Geometry: final body of the model. Coordinates: model frame, mm. A direction names the side the tool comes from. Round coordinates to 2 decimals unless told otherwise and drop trailing zeros. Loops run counter-clockwise (first coordinate to the right, second up) from the corner with the lowest first, then second, coordinate; pieces in that order, holes last. Notation, with made-up numbers: (46, -35) - (82, -35) arc R10 cw to (82, -22) - close; hole circle Ø3 at (-24.75, -37). An arc over 180 degrees is marked (long way). Answer as CSV lines item,"result".
from build123d import *

# Parameters (mm, degrees)
CROQUIS1_W              = 65
CROQUIS1_H              = 19.5
SALIENTE_EXTRUIR1_DEPTH = 16
CORTAR_EXTRUIR1_DEPTH   = 16
REDONDEO1_R             = 5
CROQUIS4_W              = 65
CROQUIS4_H              = 1.7
CORTAR_EXTRUIR2_DEPTH   = 0.57


with BuildPart() as part:
    # Croquis1 → Saliente-Extruir1 (new body)
    with BuildSketch(Plane(origin=(0, 0, 0), x_dir=(1, 0, 0), z_dir=(0, 1, 0))):
        with Locations((5.631188119, 0.14480198)):
            Rectangle(CROQUIS1_W, CROQUIS1_H)
    extrude(amount=SALIENTE_EXTRUIR1_DEPTH)

    # Croquis2 → Cortar-Extruir1 (cut)
    with BuildSketch(Plane(origin=(0, 16, 0), x_dir=(1, 0, 0), z_dir=(0, 1, 0))):
        Polygon((-26.868811881, 6.021818634), (-19.868811881, 9.89480198), (-26.868811881, 9.89480198), align=None)
        Polygon((-26.868811881, -9.60519802), (-19.868811881, -9.60519802), (-26.868811881, -5.732214674), align=None)
    extrude(amount=-CORTAR_EXTRUIR1_DEPTH, mode=Mode.SUBTRACT)

    # Redondeo1
    redondeo1_edges = [part.edges().sort_by_distance(p)[0] for p in [
        (-19.868811881, 8, -9.89480198),
        (-26.868811881, 8, -6.021818634),
        (-26.868811881, 8, 5.732214674),
        (-19.868811881, 8, 9.60519802),
    ]]
    fillet(redondeo1_edges, radius=REDONDEO1_R)

    # Croquis4 → Cortar-Extruir2 (cut)
    with BuildSketch(Plane(origin=(0, 16, 0), x_dir=(1, 0, 0), z_dir=(0, 1, 0))):
        with Locations((5.631188119, 2.223949596)):
            Rectangle(CROQUIS4_W, CROQUIS4_H)
        with Locations((5.631188119, -1.934345635)):
            Rectangle(CROQUIS4_W, CROQUIS4_H)
    extrude(amount=-CORTAR_EXTRUIR2_DEPTH, mode=Mode.SUBTRACT)


solid = part.part
(1) Section C-C (z = -6.25). Output: boundary loops of the cut face in (x, y).
Findings below:
outline,"(-25.73, 0) - (38.13, 0) - (38.13, 16) - (-25.73, 16) - close"
(2) Draft query along Z for faces 3 (the face through (5, 15.43, 2)), 4 (the face through (-22.667, 8.112, -8.347)), 5 (the face through (5, 16, 6)), 6 (the face through (-26.195, 7.888, 5.292)). Return one class per face: pulls with the +Z half, pulls with the -Z half, needs draft (parallel to the pull), parting line crosses it, or undercut.
Findings below:
face 3,"undercut"
face 4,"pulls with the -Z half"
face 5,"needs draft"
face 6,"pulls with the +Z half"
(3) Pin query (flat end, axial travel): P1, Ø0.5, axis at x = 15, z = 2, coming from the +Y side. Return the tip coordinate at first contact, or that it passes through.
Findings below:
P1,"y = 15.43"
(4) Material intervals for line 1 along Y through (x, z) = (-21, 2); line 2 along X through (y, z) = (15.5, 8.25); line 3 along X through (y, z) = (3.5, -8.5), sorted ascending.
Findings below:
line 1,"0 to 15.43"
line 2,"-22.32 to 38.13"
line 3,"-22.39 to 38.13"
(5) Section B-B (z = 6.25). Output: boundary loops of the cut face in (x, y), and give its area (3 significant figures).
Findings below:
outline,"(-25.47, 0) - (38.13, 0) - (38.13, 16) - (-25.47, 16) - close"
area,"1,020 mm2"
(6) Section A-A (y = 5). Output: boundary loops of the cut face in (x, z), and give its area (3 significant figures).
Findings below:
outline,"(-26.87, -3.07) arc R5 ccw to (-24.29, -7.45) - (-21, -9.27) arc R5 ccw to (-18.58, -9.89) - (38.13, -9.89) - (38.13, 9.61) - (-18.58, 9.61) arc R5 ccw to (-21, 8.98) - (-24.29, 7.16) arc R5 ccw to (-26.87, 2.78) - close"
area,"1,240 mm2"
(7) Access query for faces 1 (the face through (5, 16, 0)), 2 (the face through (5, 15.43, -2)). Directions: +Z, -Z, +X, -X, +Y, -Y. A direction counts if a zero-diameter tool reaches every point of the face in a straight line with its end or side. Return the directions, or none.
Findings below:
face 1,"+Z, -Z, +X, -X, +Y"
face 2,"+X, -X, +Y"
